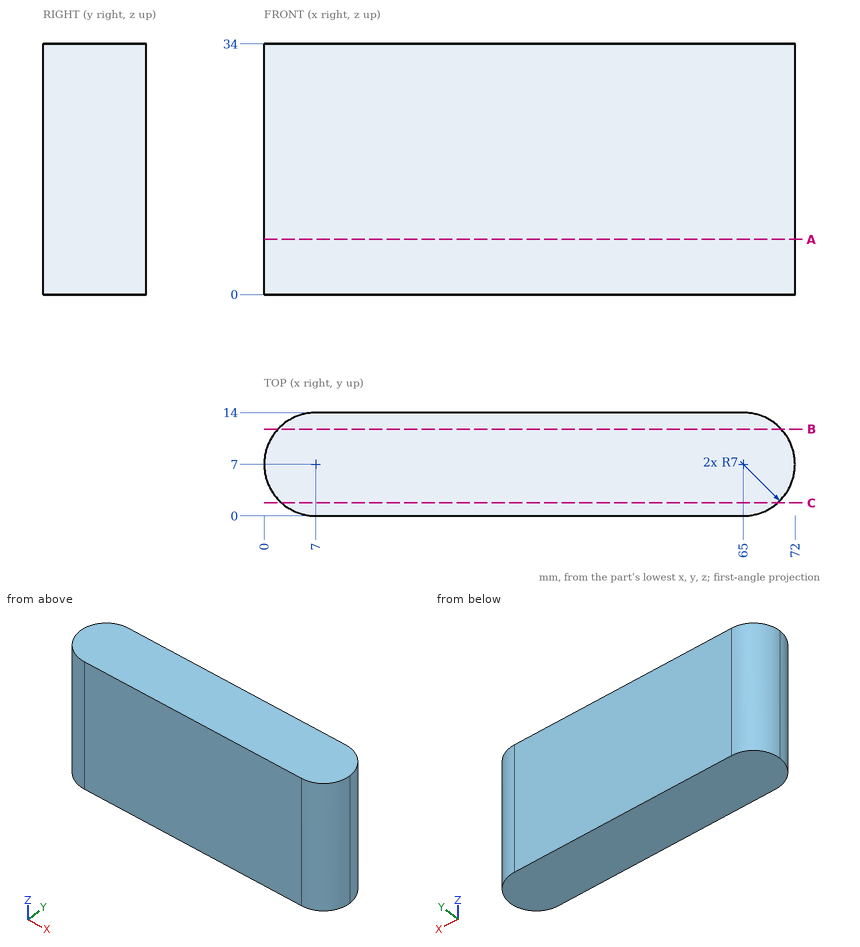
Here's the drawing with two shaded views (mm, measured from the low corner). I have some questions. Give positions to 0.01 mm unless a question says otherwise; leave off trailing zeros. Loops run counter-clockwise (first coordinate to the right, second up) from the corner with the lowest first, then second, coordinate; pieces in that order, holes last. Notation, with made-up numbers: (69.5, 4) - (123.5, 4) arc R30 cw to (123.5, 34) - close; hole circle Ø11 at (54, 52). An arc over 180 degrees is marked (long way). Answer in a Markdown table with one row per item. Add a question column.
Q1. Please list where these lines run through material, in increasing order: L1, parallel to X at y = 3, z = 19; L2, parallel to X at y = 12.5, z = 8; L3, parallel to Y at x = 4.5, z = 7.5. Write a range as from..to.
Q2. If we section it at C-C (y = 1.75): List the corners of the cut face in (x, z) for me, plus the area to 3 significant figures.
Q3. If we section it at B-B (y = 11.75): List the corners of the cut face in (x, z) for me, plus the area to 3 significant figures.
Q4. If we section it at A-A (z = 7.5): List the corners of the cut face in (x, y) for me.
The answers:
| question | item | result |
|---|---|---|
| 1 | L1 | x = 1.26..70.74 |
| 1 | L2 | x = 2.67..69.33 |
| 1 | L3 | y = 0.46..13.54 |
| 2 | outline | (2.37, 0) - (69.63, 0) - (69.63, 34) - (2.37, 34) - close |
| 2 | area | 2,290 mm^2 |
| 3 | outline | (1.86, 0) - (70.14, 0) - (70.14, 34) - (1.86, 34) - close |
| 3 | area | 2,320 mm^2 |
| 4 | outline | (0, 7) arc R7 ccw to (7, 0) - (65, 0) arc R7 ccw to (72, 7) arc R7 ccw to (65, 14) - (7, 14) arc R7 ccw to start |
